Source: three-view drawing plus pictorial views. Frame: mm from the lowest corner of the part. A direction names the side the tool comes from. Give positions to 0.01 mm unless a question says otherwise; leave off trailing zeros. Loops run counter-clockwise (first coordinate to the right, second up) from the corner with the lowest first, then second, coordinate; pieces in that order, holes last. Notation, with made-up numbers: (89, 22.5) -> (135, 22.5) arc R19 ccw to (135, 26.5) -> close; hole circle Ø9 at (2, -4.75). An arc over 180 degrees is marked (long way). Answer in a Markdown table with one row per item. Add a question column.
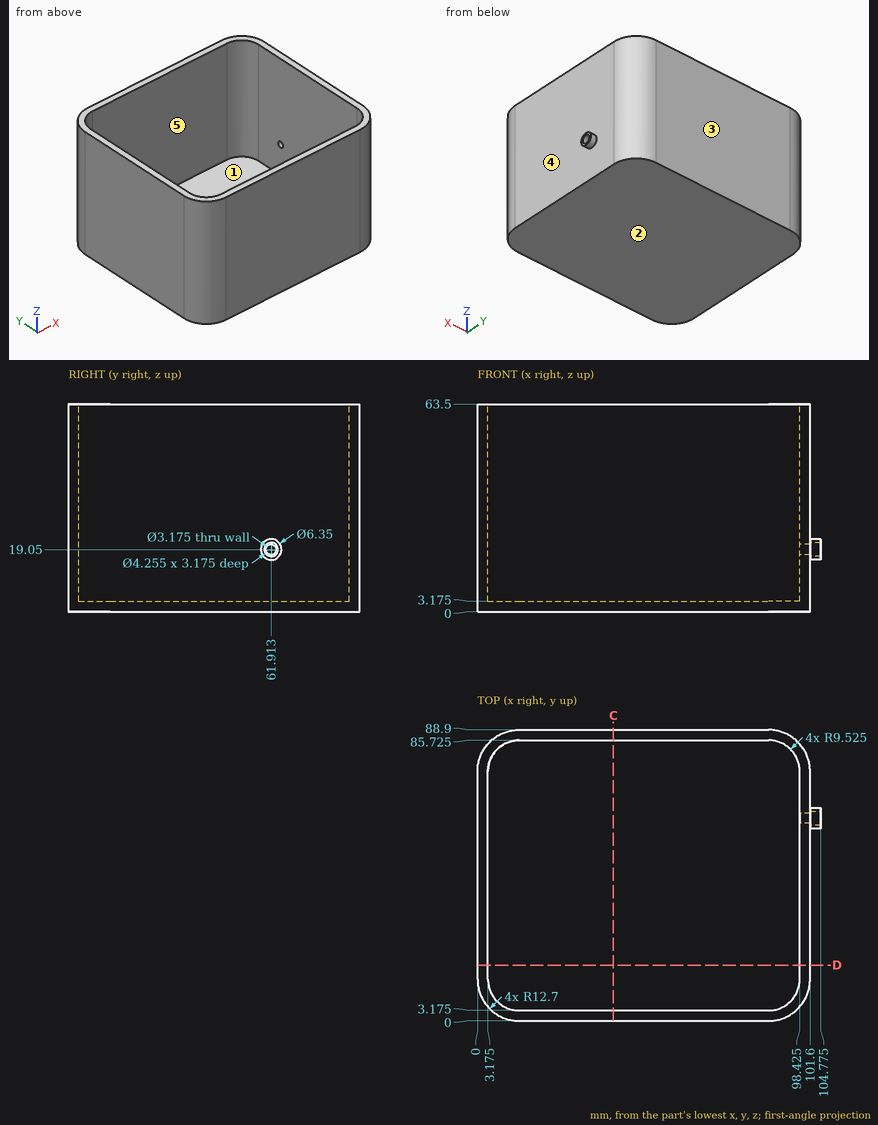
(1) Cut plane D-D on y = 17. Return the cut outline in (x, z) (1 decimal).
(2) Draft query along X for the marked faces 3, 4 and 5. Return one class per face: +X half, -X half, draft (parallel to the pull), parting line (faces both ways), or undercut.
(3) Pin query (flat end, axial travel): pin 1 Ø8 at (x, y) = (31.5, 27.5) entering from +Z (1 decimal); pin 2 Ø4 at (y, z) = (16.5, 17) entering from -X; pin 3 Ø5 at (y, z) = (72.5, 34.5) entering from +X. Return the tip coordinate at first contact, or that it passes through.
(4) Cut plane C-C on x = 41.5. Return the cut outline in (y, z) (1 decimal).
(5) Reachability of the marked faces 1 and 2 from +Z, -Z, +X, -X, +Y, -Y: full face, straight path, thin tool, end or side. Return the list, or none.
(6) Material intervals for line 1 along Y through (x, z) = (68, 50.5) (1 decimal); line 2 along X through (y, z) = (23, 21.5) (1 decimal); line 3 along Z through (x, y) = (88.5, 9.5) (1 decimal), sorted ascending. Write a range as from..to.
Answer list:
| question | item | result |
|---|---|---|
| 1 | outline | (0, 0) -> (101.6, 0) -> (101.6, 63.5) -> (98.4, 63.5) -> (98.4, 3.2) -> (3.2, 3.2) -> (3.2, 63.5) -> (0, 63.5) -> close |
| 2 | face 3 | draft |
| 2 | face 4 | +X half |
| 2 | face 5 | undercut |
| 3 | pin 1 | stops at z = 3.2 |
| 3 | pin 2 | stops at x = 0 |
| 3 | pin 3 | stops at x = 101.6 |
| 4 | outline | (0, 0) -> (88.9, 0) -> (88.9, 63.5) -> (85.7, 63.5) -> (85.7, 3.2) -> (3.2, 3.2) -> (3.2, 63.5) -> (0, 63.5) -> close |
| 5 | face 1 | +Z |
| 5 | face 2 | -Z, +X, -X, +Y, -Y |
| 6 | line 1 | y = 0..3.2, 85.7..88.9 |
| 6 | line 2 | x = 0..3.2, 98.4..101.6 |
| 6 | line 3 | z = 0..3.2 |
